Here's how the part is built. I have some questions about the finished solid (model axes, mm). Face numbers are marked on the shaded views. A direction names the side the tool comes from. Round coordinates to 2 decimals unless told otherwise and drop trailing zeros. Order: outer loops, then holes, each group sorted by start corner. A loop starts at its lowest first (then second) coordinate and runs counter-clockwise, first axis right, second up. Notation, with made-up numbers: (23, 86.5) -> (27, 86.5) arc R37 ccw to (27, 123.5) -> close; hole circle Ø3 at (-14, 29). An arc over 180 degrees is marked (long way). One line per item, written item: value.
```python
from build123d import *

# Parameters (mm, degrees)
F0_R      = 2.5
F1_DEPTH  = 5
F3_DEPTH  = 40
F4_W      = 8.75
F4_H      = 3
F4_W_2    = 4.75
F5_DEPTH  = 17
F7_DEPTH  = 2
F8_D      = 2.5
F9_R      = 5
F11_DEPTH = 2
F12_R     = 3


with BuildPart() as f1:
    # F0 (on Top) → F1 (new body)
    with BuildSketch(Plane.XY):
        with BuildLine():
            Line((10.5, 5), (4.25, -1.25))
            ThreePointArc((4.25, -1.25), (0, -5.5), (-4.25, -1.25))
            Line((-4.25, -1.25), (-10.5, 5))
            Line((-10.5, 5), (-20.5, 5))
            Line((-20.5, 5), (-20.5, -8.5))
            Line((-20.5, -8.5), (0, -8.5))
            Line((0, -8.5), (20.5, -8.5))
            Line((20.5, -8.5), (20.5, 5))
            Line((20.5, 5), (10.5, 5))
        make_face()
        with Locations((-15.5, 0)):
            Circle(F0_R, mode=Mode.SUBTRACT)
        with Locations((15.5, 0)):
            Circle(F0_R, mode=Mode.SUBTRACT)
    extrude(amount=F1_DEPTH)

    # F2 (on face) → F3 (join)
    with BuildSketch(Plane(origin=(0, 0, 0), x_dir=(1, 0, 0), z_dir=(0, 0, -1))):
        with BuildLine():
            Line((-6.25, 1.25), (-4.25, 1.25))
            ThreePointArc((-4.25, 1.25), (0, 5.5), (4.25, 1.25))
            Line((4.25, 1.25), (6.25, 1.25))
            Line((6.25, 1.25), (6.25, 8.5))
            Line((6.25, 8.5), (-6.25, 8.5))
            Line((-6.25, 8.5), (-6.25, 1.25))
        make_face()
    extrude(amount=-F3_DEPTH)

    # F4 (on face) → F5 (join)
    with BuildSketch(Plane.XY.offset(40)):
        with Locations((-10.625, -7)):
            Rectangle(F4_W, F4_H)
        Polygon((0, -5.5), (-6.25, -5.5), (-6.25, -8.5), (6.25, -8.5), (6.25, -5.5), align=None)
        with Locations((8.625, -7)):
            Rectangle(F4_W_2, F4_H)
    extrude(amount=-F5_DEPTH)

    # F6 (on face) → F7 (cut)
    with BuildSketch(Plane.XZ.offset(8.5)):
        Polygon((11, 34), (-15, 34), (-15, 23), (-6.25, 23), (6.25, 23), (11, 23), align=None)
    extrude(amount=-F7_DEPTH, mode=Mode.SUBTRACT)

    # F8 (through all)
    with Locations(Plane.XZ.offset(8.5)):
        with Locations((-11, 37), (8, 37)):
            Hole(F8_D / 2)

    # F9
    f9_edges = [f1.edges().sort_by_distance(p)[0] for p in [
        (20.5, -8.5, 2.5),
        (-20.5, 5, 2.5),
        (-20.5, -8.5, 2.5),
        (20.5, 5, 2.5),
    ]]
    fillet(f9_edges, radius=F9_R)

    # F10 (on face) → F11 (cut)
    with BuildSketch(Plane(origin=(0, 0, 0), x_dir=(1, 0, 0), z_dir=(0, 0, -1))):
        with BuildLine():
            ThreePointArc((-15.5, 8.5), (-16.7940952255, 8.3296291314), (-18, 7.8301270189))
            Line((-18, 7.8301270189), (-18, 4))
            Line((-18, 4), (-3.2403703492, 4))
            ThreePointArc((-3.2403703492, 4), (0, 5.5), (3.2403703492, 4))
            Line((3.2403703492, 4), (18, 4))
            Line((18, 4), (18, 7.8301270189))
            ThreePointArc((18, 7.8301270189), (16.7940952255, 8.3296291314), (15.5, 8.5))
            Line((15.5, 8.5), (-15.5, 8.5))
        make_face()
    extrude(amount=-F11_DEPTH, mode=Mode.SUBTRACT)

    # F12
    f12_edges = [f1.edges().sort_by_distance(p)[0] for p in [
        (6.25, -4.875, 5),
        (-6.25, -4.875, 5),
    ]]
    fillet(f12_edges, radius=F12_R)


solid = f1.part
```
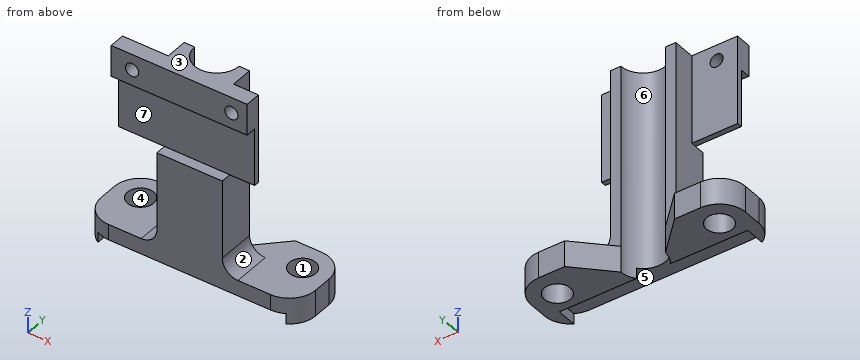
Q1. I need wall thicknesses on line 1 along Z through (x, y) = (-14.5, -7.5); line 2 along Z through (x, y) = (-2, -7.75); line 3 along Y through (x, z) = (-15.5, 3.1). Which ranges of each line are inside material? Lowest first, please.
Answers:
line 1: 2 to 5, 34 to 40
line 2: 2 to 23, 34 to 40
line 3: -8.5 to -2.5, 2.5 to 5
Q2. I want a section at C-C on y = 3.5. Write out the boundary of the cut face in (x, z).
Answers:
outline: (-19.07, 0) -> (-9, 0) -> (-9, 5) -> (-19.07, 5) -> close; (9, 0) -> (19.07, 0) -> (19.07, 5) -> (9, 5) -> close
Q3. If we mould it in two halves opening along X, with no side actions, what happens to the marked faces 1, 2, 3 and 4? For each: pulls with the +X half, pulls with the -X half, needs draft (parallel to the pull), parting line crosses it, or undercut.
Answers:
face 1: undercut
face 2: pulls with the +X half
face 3: needs draft
face 4: undercut
Q4. I want a section at D-D on y = -7. Write out the boundary of the cut face in (x, z).
Answers:
outline: (-19.07, 0) -> (-18, 0) -> (-18, 2) -> (18, 2) -> (18, 0) -> (19.07, 0) -> (19.07, 5) -> (9.25, 5) arc R3 cw to (6.25, 8) -> (6.25, 23) -> (-6.25, 23) -> (-6.25, 8) arc R3 cw to (-9.25, 5) -> (-19.07, 5) -> close; (-15, 34) -> (11, 34) -> (11, 40) -> (-15, 40) -> close; hole circle Ø2.5 at (-11, 37); hole circle Ø2.5 at (8, 37)
Q5. For P1, Ø6, axis at y = -4, z = 14, coming from the -X side; P2, Ø3, axis at y = 0, z = 28, coming from the +X side; P3, Ø3.5, axis at x = -5.5, z = 26.5, coming from the -Y side, each with a flat end and sliding along its axis, tell me the tip position at first contact or that it passes through.
Answers:
P1: x = -6.25
P2: x = 6.25
P3: y = -6.5
Q6. I want a section at B-B on z = 4.5. Write out the boundary of the cut face in (x, y).
Answers:
outline: (-20.5, -3.5) arc R5 ccw to (-15.5, -8.5) -> (15.5, -8.5) arc R5 ccw to (20.5, -3.5) -> (20.5, 0) arc R5 ccw to (15.5, 5) -> (10.5, 5) -> (4.25, -1.25) arc R4.25 cw to (-4.25, -1.25) -> (-10.5, 5) -> (-15.5, 5) arc R5 ccw to (-20.5, 0) -> close; hole circle Ø5 at (-15.5, 0); hole circle Ø5 at (15.5, 0)
Q7. I want a section at A-A on z = 37. Write out the boundary of the cut face in (x, y).
Answers:
outline: (-15, -8.5) -> (-12.25, -8.5) -> (-12.25, -5.5) -> (-15, -5.5) -> close; (-9.75, -8.5) -> (6.75, -8.5) -> (6.75, -5.5) -> (6.25, -5.5) -> (6.25, -1.25) -> (4.25, -1.25) arc R4.25 cw to (-4.25, -1.25) -> (-6.25, -1.25) -> (-6.25, -5.5) -> (-9.75, -5.5) -> close; (9.25, -8.5) -> (11, -8.5) -> (11, -5.5) -> (9.25, -5.5) -> close
Q8. Which directions (+Z, -Z, +X, -X, +Y, -Y) give clear straight access to the entire face, cutting with the end or side of a thin tool? Please do the marked faces 5, 6 and 7.
Answers:
face 5: -Z, -Y
face 6: +Z, -Z, +Y
face 7: +X, -X, -Y
